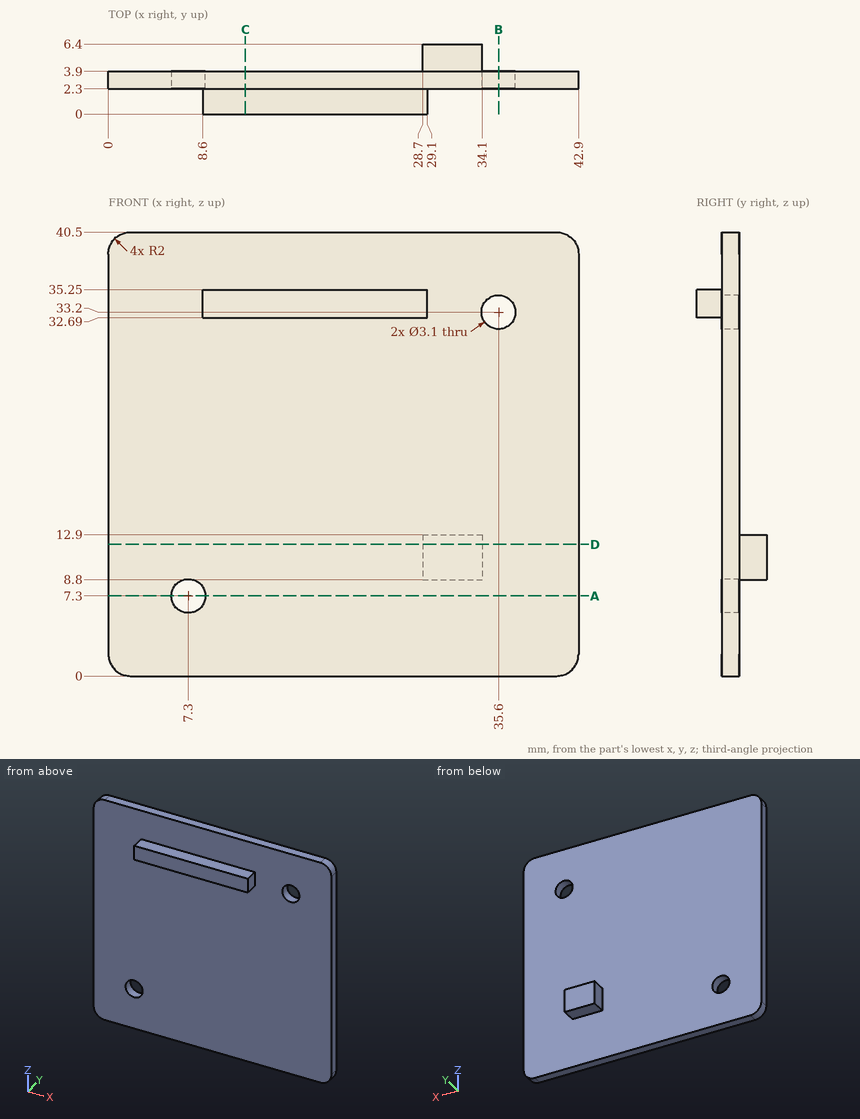
Geometry check sheet. Reference: drawing and pictorial views, mm from the part's lowest x, y, z. Coordinates: 2 decimals unless noted, no trailing zeros. Order: outer loops, then holes, each group sorted by start corner. A loop starts at its lowest first (then second) coordinate and runs counter-clockwise, first axis right, second up. Notation, with made-up numbers: M 40.5,59.25 L 85.5,59.25 A13 cw 85.5,68.25 Z; hole C 9.25,18.5 d3. An arc over 180 degrees is marked long. Write each question's results on one line, items separated by ' | '. Start each with the question number.
1. Cross-section at A-A on z = 7.3. Record the cut outline in (x, y), and give its area (3 significant figures).
2. Material ranges on probe 1 along Z at (x, y) = (7.3, 3.3); probe 2 along X at (y, z) = (2.8, 33.2); probe 3 along Z at (x, y) = (35.6, 3.45), recorded low to high.
3. Cross-section at D-D on z = 12. Record the cut outline in (x, y).
4. Go/stop test with flat-tipped pins: P1, Ø1.8, axis at y = 1, z = 34.5, coming from the +X side; P2, Ø2, axis at y = 5.5, z = 12, coming from the +X side; P3, Ø0.8, axis at y = 5, z = 11, coming from the -X side. Record where each tip stops, or that it passes through.
5. Cross-section at C-C on x = 12.5. Record the cut outline in (y, z).
6. Cross-section at B-B on x = 35.6. Record the cut outline in (y, z).
Checks:
1) outline: M 0,2.3 L 5.75,2.3 L 5.75,3.9 L 0,3.9 Z; M 8.85,2.3 L 42.9,2.3 L 42.9,3.9 L 8.85,3.9 Z | area: 63.7 mm²
2) probe 1: z = 0 to 5.75, 8.85 to 40.5 | probe 2: x = 0 to 34.05, 37.15 to 42.9 | probe 3: z = 0 to 31.65, 34.75 to 40.5
3) outline: M 0,2.3 L 42.9,2.3 L 42.9,3.9 L 34.1,3.9 L 34.1,6.4 L 28.7,6.4 L 28.7,3.9 L 0,3.9 Z
4) P1: stops at x = 29.1 | P2: stops at x = 34.1 | P3: stops at x = 28.7
5) outline: M 0,32.69 L 2.3,32.69 L 2.3,0 L 3.9,0 L 3.9,40.5 L 2.3,40.5 L 2.3,35.25 L 0,35.25 Z
6) outline: M 2.3,0 L 3.9,0 L 3.9,31.65 L 2.3,31.65 Z; M 2.3,34.75 L 3.9,34.75 L 3.9,40.5 L 2.3,40.5 Z
